Here's how the part is built. I have some questions about the finished solid (model axes, mm). Face numbers are marked on the shaded views. A direction names the side the tool comes from. Give positions to 0.01 mm unless a question says otherwise; leave off trailing zeros. Order: outer loops, then holes, each group sorted by start corner. A loop starts at its lowest first (then second) coordinate and runs counter-clockwise, first axis right, second up. Notation, with made-up numbers: (68, -32.5) -> (120, -32.5) arc R15 ccw to (120, -26.5) -> close; hole circle Ø6 at (20, 20). An arc over 180 degrees is marked (long way). Write each question's results on one line, items separated by ' | '. Start each with the question number.
Q1. Imagine slicing it at B-B, the plane y = 7.5. Please give me the cut outline in (x, z), then the cut area to 3 significant figures.
Q2. Imagine slicing it at D-D, the plane x = -63. Please give me the cut outline in (y, z), then the cut area to 3 significant figures.
Q3. Imagine slicing it at A-A, the plane z = -12.5. Please give me the cut outline in (x, y), then the cut area to 3 significant figures.
Q4. Thinking about a two-plate mould opening in Y: for the marked faces 1, 2, 3 and 4, which applies, pulls with the +Y half, pulls with the -Y half, needs draft (parallel to the pull), parting line crosses it, or undercut?
Q5. For the marked faces 5, 6, 7 and 8, which set-ups out of +Z, -Z, +X, -X, +Y, -Y let a thin tool reach every point of the face, with its end or its side?
Q6. I'm going to push flat-ended pins straight in: pin 1 (6.5 mm diameter, centred on x = -27.59, z = -13.49, fed in from +Y); pin 2 (5 mm diameter, centred on x = -42.5, y = 22.5, fed in from +Z); pin 3 (10 mm diameter, centred on x = -43.5, y = 45, fed in from -Z); pin 4 (1.5 mm diameter, centred on x = -34.5, z = -16.5, fed in from -Y). Where does each tip first touch, or does it pass through?
Q7. I need wall thicknesses on line 1 along Z through (x, y) = (-36.5, 4); line 2 along Y through (x, z) = (-56, -29); line 3 along X through (y, z) = (23, -14.5). Which ranges of each line are inside material? Lowest first, please. Write a range as [from, to].
Q8. Imagine slicing it at C-C, the plane z = -34. Please give me the cut outline in (x, y).
Solid Edge part; units mm, degrees
sketch "Sketch1" plane through (10.8674, 0, 10.8674) normal (0, -1, 0) x (1, 0, 0)
  line L0 (-78.9583, -8.8575) -> (-28.1583, -8.8575)
  line L1 (-28.1583, -8.8575) -> (-28.1583, -28.8575)
  line L2 (-28.1583, -28.8575) -> (-44.7332, -59.9604)
  arc A0 (-62.3834, -59.9604) -> (-44.7332, -59.9604) centre (-53.5583, -55.2575) ccw
  line L3 (-62.3834, -59.9604) -> (-78.9583, -28.8575)
  line L4 (-78.9583, -28.8575) -> (-78.9583, -8.8575)
  dimension "D1" = 78.9583
  dimension "D2" = 28.1583
  dimension "D3" = 28.1583
extrude "Protrusion1" add sketch "Sketch1" against normal blind 3
sketch "Sketch2" plane through (-42.691, 1.5, 2.0099) normal (0, 0, 1) x (-1, 0, 0)
  line L0 (25.4, 1.5) -> (-25.4, 1.5)
  line L1 (-25.4, -18.5) -> (-25.4, 1.5)
  line L2 (-25.4, -18.5) -> (-14.7727, -44.9193)
  line L3 (25.4, -18.5) -> (14.7727, -44.9193)
  line L4 (25.4, -18.5) -> (25.4, 1.5)
  arc A0 (-14.7727, -44.9193) -> (14.7727, -44.9193) centre (0, -38.977) ccw
  dimension "D1" = 25.4
extrude "Horizontal" add sketch "Sketch2" against normal blind 3
sketch "Sketch3" plane through (-42.691, 56.4, 2.0099) normal (1, 0, 0) x (0, -0.9984256, -0.0560913)
  line L0 (53.4842, 0) -> (55.7279, 39.937)
  line L1 (55.7279, 39.937) -> (13.5472, 2.2437)
  line L2 (53.4842, 0) -> (13.5472, 2.2437)
  dimension "D1" = 53.4842
extrude "Support" add sketch "Sketch3" along normal mid plane 3
sketch "Sketch4" plane through (-42.691, 29.7, -0.9901) normal (0, 0, -1) x (-1, 0, 0)
  circle A0 centre (0, 10.777) radius 10
extrude "Outlet" add sketch "Sketch4" along normal blind 15
sketch "Sketch5" plane through (-42.691, 40.477, -15.9901) normal (0, 0, -1) x (0, -1, 0)
  circle A0 centre (0, 0) radius 2.9378
extrude "OutletThin" add sketch "Sketch5" along normal blind 10
sketch "Sketch6" plane through (-42.691, 40.477, -25.9901) normal (0, 0, -1) x (0, -1, 0)
  circle A0 centre (0, 0) radius 4.5
extrude "OutletValve" add sketch "Sketch6" along normal blind 5 draft 20
sketch "Sketch7" plane through (-42.691, 28.2, 2.0099) normal (0, 0, 1) x (-1, 0, 0)
  circle A0 centre (0, -12.277) radius 10
extrude "Inlet" add sketch "Sketch7" along normal blind 15
sketch "Sketch8" plane through (-42.691, 30.477, 17.0099) normal (-1, 0, 0) x (0, 1, 0)
  line L0 (19, 3) -> (22, 3)
  line L1 (22, 3) -> (22, 6)
  line L2 (22, 6) -> (19, 6)
  line L3 (19, 6) -> (19, 3)
  dimension "D1" = 22
  dimension "D2" = 22
revolve "RevolvedCutout1" cut sketch "Sketch8" angle 360 about axis through (-42.691, 40.477, -30.9901) along (0, 0, 1)
chamfer "InletChamfer" distance 1 angle 45 1 edges at (-32.691, 40.477, 17.0099)
hole "Hole1" at (-57.791, 0, -13.4901) direction (0, 1, 0) diameter 4.826 end up to next
hole "Hole2" at (-27.591, 0, -13.4901) direction (0, 1, 0) diameter 4.826 end up to next
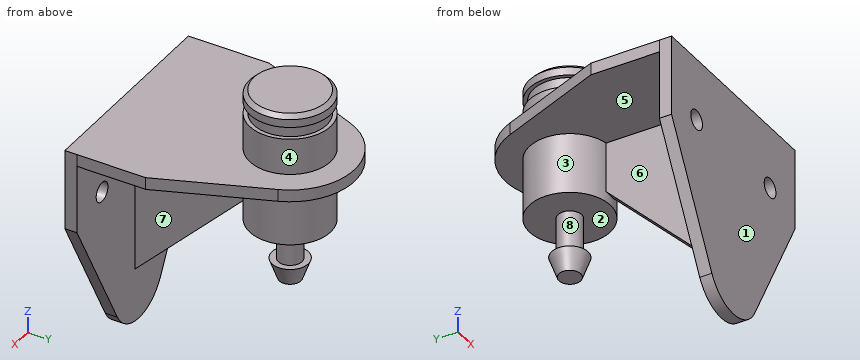
Geometry check:
1) outline: (-68.09, -0.99) -> (-44.19, -0.99) -> (-44.19, -36.49) -> (-41.19, -36.49) -> (-41.19, -0.99) -> (-17.29, -0.99) -> (-17.29, 2.01) -> (-68.09, 2.01) -> close | area: 259 mm²
2) outline: (0, -27.54) -> (3, -27.54) -> (3, -0.99) -> (32.66, -0.99) -> (32.66, 2.01) -> (0, 2.01) -> close | area: 178 mm²
3) outline: (-68.09, 0) -> (-59.99, 0) -> (-59.99, 3) -> (-68.09, 3) -> close; (-55.59, 0) -> (-29.79, 0) -> (-29.79, 3) -> (-41.19, 3) -> (-41.19, 30.59) arc R10 ccw (long way) to (-44.19, 30.59) -> (-44.19, 3) -> (-55.59, 3) -> close; (-25.39, 0) -> (-17.29, 0) -> (-17.29, 3) -> (-25.39, 3) -> close | area: 523 mm²
4) face 1: pulls with the -Y half | face 2: undercut | face 3: undercut | face 4: parting line crosses it
5) face 5: -Z | face 6: -Z, -X | face 7: -Z, +X | face 8: none
6) pin 1: y = 3 | pin 2: z = 2.01 | pin 3: z = -30.99 | pin 4: y = 0
7) line 1: [-0.99, 2.01] | line 2: [0, 3] | line 3: [-44.19, -41.19]
8) outline: (-59.56, 0) -> (-25.82, 0) -> (-25.82, 3) -> (-41.19, 3) -> (-41.19, 9.99) -> (-44.19, 9.99) -> (-44.19, 3) -> (-59.56, 3) -> close
